from build123d import *

# Parameters (mm, degrees)
F0_R     = 9
F1_DEPTH = 12.5
F2_R     = 5
F3_DEPTH = 12
F4_R     = 2.5
F5_DEPTH = 13
F7_R     = 1
F8_DEPTH = 9


with BuildPart() as f1:
    # F0 (on Right) → F1 (new body, symmetric)
    with BuildSketch(Plane.YZ):
        Circle(F0_R)
    extrude(amount=F1_DEPTH, both=True)

    # F2 (on face) → F3 (cut)
    with BuildSketch(Plane.YZ.offset(12.5)):
        Circle(F2_R)
    extrude(amount=-F3_DEPTH, mode=Mode.SUBTRACT)

    # F4 (on face) → F5 (cut)
    with BuildSketch(Plane(origin=(-12.5, 0, 0), x_dir=(0, -1, 0), z_dir=(-1, 0, 0))):
        Circle(F4_R)
    extrude(amount=-F5_DEPTH, mode=Mode.SUBTRACT)

    # F7 (on offset) → F8 (cut)
    with BuildSketch(Plane.XZ.offset(9)):
        with Locations((7.094594, 0)):
            Circle(F7_R)
        with Locations((-7.094594, 0)):
            Circle(F7_R)
    extrude(amount=-F8_DEPTH, mode=Mode.SUBTRACT)


solid = f1.part
Input: part model. Units: mm. Frame: model coordinates. A direction names the side the tool comes from. Coordinates: 2 decimals unless noted, no trailing zeros. Order: outer loops, then holes, each group sorted by start corner. A loop starts at its lowest first (then second) coordinate and runs counter-clockwise, first axis right, second up. Notation, with made-up numbers: M 72,38.5 L 84,38.5 A22 ccw 84,77.5 Z; hole C 66,14.25 d7. An arc over 180 degrees is marked long. One line per question, with ' | ' between items.
Item 1: Section B-B (z = 0). Output: boundary loops of the cut face in (x, y), then the cut area to 3 significant figures.
Geometry results:
outline: M -12.5,-9 L -8.09,-9 L -8.09,-2.5 L -12.5,-2.5 Z; M -12.5,2.5 L 0.5,2.5 L 0.5,5 L 12.5,5 L 12.5,9 L -12.5,9 Z; M -6.09,-9 L 6.09,-9 L 6.09,-5 L 0.5,-5 L 0.5,-2.5 L -6.09,-2.5 Z; M 8.09,-9 L 12.5,-9 L 12.5,-5 L 8.09,-5 Z | area: 244 mm^2
Item 2: Section C-C (y = 4.25). Output: boundary loops of the cut face in (x, z), then the cut area to 3 significant figures.
Geometry results:
outline: M -12.5,-7.93 L 12.5,-7.93 L 12.5,-2.63 L 0.5,-2.63 L 0.5,2.63 L 12.5,2.63 L 12.5,7.93 L -12.5,7.93 Z | area: 333 mm^2
Item 3: Section A-A (y = 0). Output: boundary loops of the cut face in (x, z).
Geometry results:
outline: M -12.5,-9 L 12.5,-9 L 12.5,-5 L 0.5,-5 L 0.5,-2.5 L -12.5,-2.5 Z; M -12.5,2.5 L 0.5,2.5 L 0.5,5 L 12.5,5 L 12.5,9 L -12.5,9 Z
Item 4: Section D-D (x = -1.75). Output: boundary loops of the cut face in (y, z).
Geometry results:
outline: C 0,0 d18; hole C 0,0 d5
Item 5: Draft query along X for faces 4 (the cylindrical face through (-6.1, 2, -1.5)), 5 (the flat face through (0.5, 2, -2)), 6 (the cylindrical face through (-8.094, -5.693, 0.044)). Return one class per face: released by +X, released by -X, zero draft, split by the parting line, or undercut.
Geometry results:
face 4: zero draft | face 5: released by +X | face 6: undercut
Item 6: Pin query (flat end, axial travel): pin 1 (4 mm diameter, centred on x = -3, y = -5, fed in from +Z); pin 2 (4 mm diameter, centred on y = 0, z = 0, fed in from +X); pin 3 (8 mm diameter, centred on x = -7.5, y = 7, fed in from -Z); pin 4 (4 mm diameter, centred on x = 3, z = 3.5, fed in from -Y). Return the tip coordinate at first contact, or that it passes through.
Geometry results:
pin 1: stops at z = 8.49 | pin 2: passes through | pin 3: stops at z = -8.49 | pin 4: stops at y = -8.87
Item 7: Ray query, line 1 along Z through (x, y) = (-7.75, 0); line 2 along Z through (x, y) = (-1.5, 2.25); line 3 along Y through (x, z) = (-8, 2). Return the intervals inside material, ascending.
Geometry results:
line 1: z = -9 to -2.5, 2.5 to 9 | line 2: z = -8.71 to -1.09, 1.09 to 8.71 | line 3: y = -8.77 to -1.5, 1.5 to 8.77
Item 8: Reachability of faces 1 (the cylindrical face through (8.02, -6.98, -0.38)), 2 (the cylindrical face through (6.58, 4.77, 1.5)), 3 (the cylindrical face through (0.175, -1.172, 8.923)) from +Z, -Z, +X, -X, +Y, -Y: full face, straight path, thin tool, end or side. Return the list, or none.
Geometry results:
face 1: -Y | face 2: +X | face 3: +X, -X
